Verification items for this drawing (mm, ordinates from the low corner). Coordinates: 2 decimals unless noted, no trailing zeros. Loops run counter-clockwise (first coordinate to the right, second up) from the corner with the lowest first, then second, coordinate; pieces in that order, holes last. Notation, with made-up numbers: (36, 51) -> (78, 51) arc R34 cw to (78, 88) -> close; hole circle Ø3 at (-21.75, 33.5). An arc over 180 degrees is marked (long way). Write item = value, one per line.
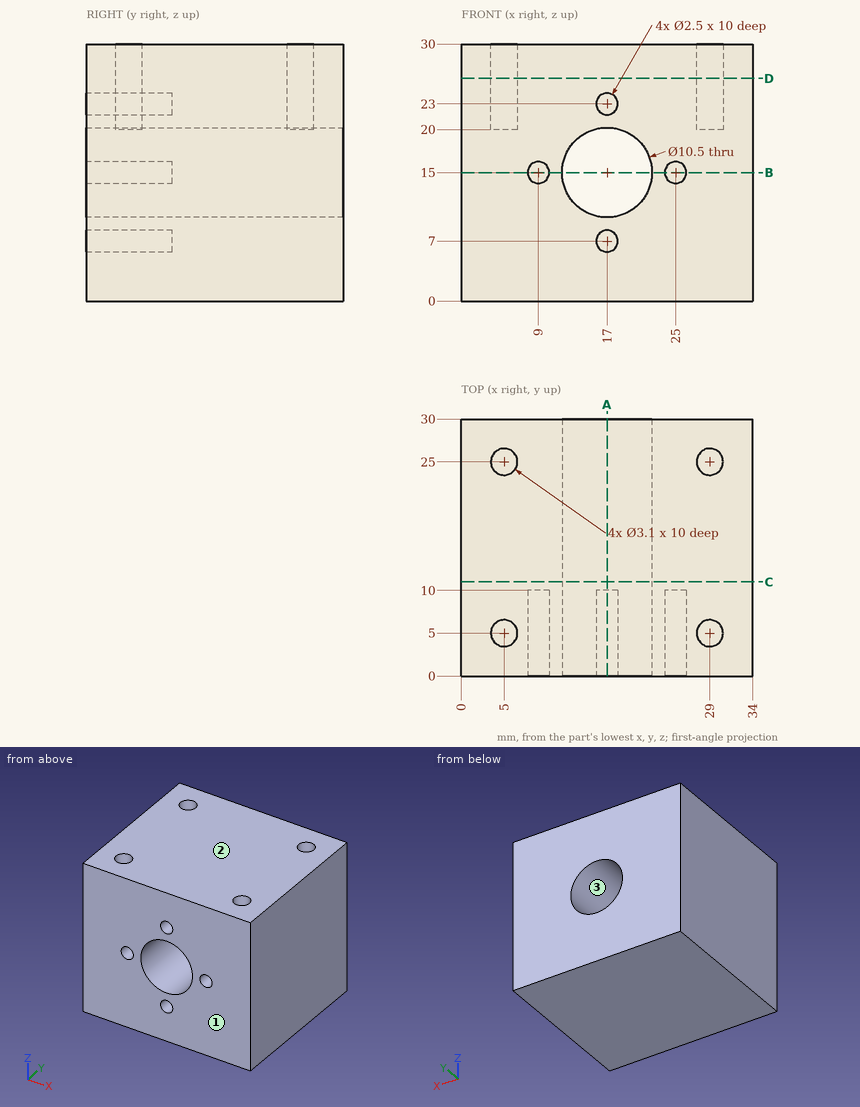
1) Sectioned sample at C-C, the plane y = 11. Record the cut outline in (x, z).
Ans:
outline = (0, 0) -> (34, 0) -> (34, 30) -> (0, 30) -> close; hole circle Ø10.5 at (17, 15)
2) Release check for a two-part mould opening along Z. For the marked faces 1, 2 and 3 record: pulls with the +Z half, pulls with the -Z half, needs draft (parallel to the pull), parting line crosses it, or undercut.
Ans:
face_1 = needs draft
face_2 = pulls with the +Z half
face_3 = undercut
3) Sectioned sample at B-B, the plane z = 15. Record the cut outline in (x, y), plus the area to 3 significant figures.
Ans:
outline = (0, 0) -> (7.75, 0) -> (7.75, 10) -> (10.25, 10) -> (10.25, 0) -> (11.75, 0) -> (11.75, 30) -> (0, 30) -> close; (22.25, 0) -> (23.75, 0) -> (23.75, 10) -> (26.25, 10) -> (26.25, 0) -> (34, 0) -> (34, 30) -> (22.25, 30) -> close
area = 655 mm2
4) Sectioned sample at D-D, the plane z = 26. Record the cut outline in (x, y).
Ans:
outline = (0, 0) -> (34, 0) -> (34, 30) -> (0, 30) -> close; hole circle Ø3.1 at (5, 5); hole circle Ø3.1 at (5, 25); hole circle Ø3.1 at (29, 5); hole circle Ø3.1 at (29, 25)
5) Depth check by flat-ended pin: pin 1 Ø1.6 at (x, y) = (29, 25.5) entering from +Z; pin 2 Ø2.5 at (x, y) = (5.5, 24) entering from +Z; pin 3 Ø1.2 at (x, z) = (17, 22.5) entering from -Y. Enter the tip coordinate at first touch or a pass-through.
Ans:
pin_1 = 20
pin_2 = 30
pin_3 = 10
6) Material ranges on line 1 (Y direction, x = 29, z = 25); line 2 (Z direction, x = 18, y = 6.5); line 3 (X direction, y = 8.75, z = 16), recorded low to high.
Ans:
line_1 = 0 to 3.45, 6.55 to 23.45, 26.55 to 30
line_2 = 0 to 6.25, 7.75 to 9.85, 20.15 to 22.25, 23.75 to 30
line_3 = 0 to 8.25, 9.75 to 11.85, 22.15 to 24.25, 25.75 to 34
7) Sectioned sample at A-A, the plane x = 17. Record the cut outline in (y, z).
Ans:
outline = (0, 0) -> (30, 0) -> (30, 9.75) -> (0, 9.75) -> (0, 8.25) -> (10, 8.25) -> (10, 5.75) -> (0, 5.75) -> close; (0, 20.25) -> (30, 20.25) -> (30, 30) -> (0, 30) -> (0, 24.25) -> (10, 24.25) -> (10, 21.75) -> (0, 21.75) -> close
